Design review of the part built by this model. Coordinates are the model's own, in mm. A direction names the side the tool comes from. Coordinates: 2 decimals unless noted, no trailing zeros. Loops run counter-clockwise (first coordinate to the right, second up) from the corner with the lowest first, then second, coordinate; pieces in that order, holes last. Notation, with made-up numbers: (-26, 82) -> (2, 82) arc R6 ccw to (2, 87) -> close; hole circle Ø4 at (79.25, 69). An arc over 180 degrees is marked (long way). Use one line per item in the form item = value. Start each with the question number.
1. Machinability: for faces 1 (the face through (1.48, 100.05, 1.43)), 2 (the face through (0.057, 50.779, -0.52)), which of the approach directions +Z, -Z, +X, -X, +Y, -Y give a long, thin tool a straight path to every point of the face, cutting with its end or side? Answer none if there is none.
2. Consider section C-C (y = 100.5). State the section outline as (x, z) points, then the cut area to 3 significant figures.
3. Consider section A-A (z = 0). State the section outline as (x, y) points, then the cut area to 3 significant figures.
4. The part is to be moulded in two halves that separate along Y. For faces 3 (the face through (2, 0, 0)), 4 (the face through (1.479, 12.075, 1.386)), 5 (the face through (2, 103, 0)), say which applies: released by +Y, released by -Y, zero draft, split by the parting line, or undercut.
5. Consider section B-B (y = 63.5). State the section outline as (x, z) points.
6. Wall thickness on line 1 (Y direction, x = 2.15, z = 0); line 2 (Y direction, x = 1.5, z = -0.55); line 3 (Z direction, x = 2.6, y = 69.5): over which ranges is each line inside the solid? List them lowest first. Write a range as from..to.
7. For pin 1 (2.5 mm diameter, centred on y = 2.5, z = 0, fed in from -X); pin 2 (1 mm diameter, centred on x = 3, y = 10.5, fed in from +Z), all flat-tipped, find the tip position at first contact; note any pin that passes through.
from build123d import *

# Parameters (mm, degrees)
SZKIC5_R                    = 2.4
DODANIE_WYCI_GNI_CIE2_DEPTH = 103
SZKIC6_R                    = 1.5
WYTNIJ_WYCI_GNI_CIE1_DEPTH  = 3


with BuildPart() as part:
    # Szkic5 → Dodanie-wyciągnięcie2 (new body)
    with BuildSketch(Plane(origin=(0, 0, 0), x_dir=(1, 0, 0), z_dir=(0, 1, 0))):
        with Locations(Location((2.4, 0, 0), (0, 0, 270))):
            Circle(SZKIC5_R)
    extrude(amount=DODANIE_WYCI_GNI_CIE2_DEPTH)

    # Szkic6 → Wytnij-wyciągnięcie1 (cut)
    with BuildSketch(Plane(origin=(0, 0, 0), x_dir=(0, 0, -1), z_dir=(1, 0, 0))):
        with Locations(Location((0, 2.5, 0), (0, 0, 180))):
            Circle(SZKIC6_R)
        with Locations(Location((0, 11.5, 0), (0, 0, 180))):
            Circle(SZKIC6_R)
        with Locations(Location((0, 91.5, 0), (0, 0, 180))):
            Circle(SZKIC6_R)
        with Locations(Location((0, 100.5, 0), (0, 0, 180))):
            Circle(SZKIC6_R)
    extrude(amount=WYTNIJ_WYCI_GNI_CIE1_DEPTH, mode=Mode.SUBTRACT)


solid = part.part
Geometry check:
q1.face_1 = -X
q1.face_2 = +Y, -Y
q2.outline = (0.53, -1.5) arc R2.4 ccw (long way) to (0.53, 1.5) -> (3, 1.5) -> (3, -1.5) -> close
q2.area = 9.60 mm²
q3.outline = (0, 0) -> (4.8, 0) -> (4.8, 103) -> (0, 103) -> (0, 102) -> (3, 102) -> (3, 99) -> (0, 99) -> (0, 93) -> (3, 93) -> (3, 90) -> (0, 90) -> (0, 13) -> (3, 13) -> (3, 10) -> (0, 10) -> (0, 4) -> (3, 4) -> (3, 1) -> (0, 1) -> close
q3.area = 458 mm²
q4.face_3 = released by -Y
q4.face_4 = undercut
q4.face_5 = released by +Y
q5.outline = circle Ø4.8 at (2.4, 0)
q6.line_1 = 0..1, 4..10, 13..90, 93..99, 102..103
q6.line_2 = 0..1.1, 3.9..10.1, 12.9..90.1, 92.9..99.1, 101.9..103
q6.line_3 = -2.39..2.39
q7.pin_1 = 3
q7.pin_2 = 2.4
